The model under review builds one solid part; all positions refer to its coordinate system, in mm. Face numbers are marked on the shaded views. A direction names the side the tool comes from. Give positions to 0.01 mm unless a question says otherwise; leave off trailing zeros. Write each loop counter-clockwise with the first axis right and the second up, starting at its lowest first coordinate (ties: lowest second). Pieces come first, ordered by that corner, then holes. Notation, with made-up numbers: (64.25, 29.5) - (104.25, 29.5) arc R14 ccw to (104.25, 38.5) - close; hole circle Ø5 at (52, -27.5). An arc over 180 degrees is marked (long way). One line per question, with ' | ' between items. Start each with the question number.
```python
from build123d import *

# Parameters (mm, degrees)
SZKIC1_W                    = 40
SZKIC1_H                    = 20
SZKIC1_R                    = 2.25
DODANIE_WYCI_GNI_CIE1_DEPTH = 2
SZKIC3_W                    = 22
SZKIC3_H                    = 20
DODANIE_WYCI_GNI_CIE3_DEPTH = 3
ZAOKR_GLENIE1_R             = 3


with BuildPart() as part:
    # Szkic1 → Dodanie-wyciągnięcie1 (new body)
    with BuildSketch(Plane.XY):
        with Locations((0.494567618, 0.286392586)):
            Rectangle(SZKIC1_W, SZKIC1_H)
        with Locations((-9.505432382, 5.286392586)):
            Circle(SZKIC1_R, mode=Mode.SUBTRACT)
        with Locations((-9.505432382, -4.713607414)):
            Circle(SZKIC1_R, mode=Mode.SUBTRACT)
    extrude(amount=DODANIE_WYCI_GNI_CIE1_DEPTH)

    # Szkic3 → Dodanie-wyciągnięcie3 (add)
    with BuildSketch(Plane.XY.offset(2)):
        with Locations((9.494567618, 0.286392586)):
            Rectangle(SZKIC3_W, SZKIC3_H)
    extrude(amount=DODANIE_WYCI_GNI_CIE3_DEPTH)

    # Zaokrąglenie1
    zaokr_glenie1_edges = [part.edges().sort_by_distance(p)[0] for p in [
        (20.494567618, -9.713607414, 2.5),
        (-19.505432382, -9.713607414, 1),
        (-19.505432382, 10.286392586, 1),
        (20.494567618, 10.286392586, 2.5),
        (-1.505432382, 10.286392586, 3.5),
        (-1.505432382, -9.713607414, 3.5),
    ]]
    fillet(zaokr_glenie1_edges, radius=ZAOKR_GLENIE1_R)


solid = part.part
```
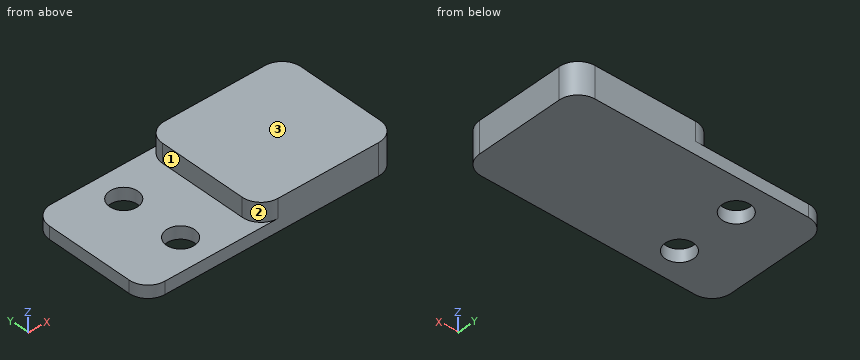
Item 1: Machinability: for the marked faces 1, 2 and 3, which of the approach directions +Z, -Z, +X, -X, +Y, -Y give a long, thin tool a straight path to every point of the face, cutting with its end or side? Answer none if there is none.
Item 2: Clearance check with flat-ended pins moving along their axes: P1, Ø10, axis at x = -8.5, y = 1, coming from the +Z side; P2, Ø2.5, axis at x = -9.51, y = 5.29, coming from the -Z side. State where each tip first meets the part, or that it passes through.
Item 3: Take a section at A-A (y = 5.75). Give the boundary of the cut face in (x, z), plus the area to 3 significant figures.
Item 4: Take a section at D-D (y = -1.5). Give the boundary of the cut face in (x, z).
Item 5: Take a section at C-C (x = -9). Give the boundary of the cut face in (y, z).
Item 6: Take a section at B-B (z = 1.25). Give the boundary of the cut face in (x, y).
Item 7: For probe 1 along Y at (x, z) = (-9, 1.25); probe 2 along Z at (x, y) = (-3, 3.75); probe 3 along X at (y, z) = (1.75, 3.05), list the stretches that pass through material, from the lowest coordinate up.
Check sheet entries:
1) face 1: +Z, -X, +Y, -Y | face 2: +Z, -X, -Y | face 3: +Z, +X, -X, +Y, -Y
2) P1: stops at z = 2 | P2: passes through
3) outline: (-19.51, 0) - (-11.71, 0) - (-11.71, 2) - (-19.51, 2) - close; (-7.3, 0) - (20.49, 0) - (20.49, 5) - (-1.51, 5) - (-1.51, 2) - (-7.3, 2) - close | area: 137 mm^2
4) outline: (-19.51, 0) - (20.49, 0) - (20.49, 5) - (-1.51, 5) - (-1.51, 2) - (-19.51, 2) - close
5) outline: (-9.71, 0) - (-6.91, 0) - (-6.91, 2) - (-9.71, 2) - close; (-2.52, 0) - (3.09, 0) - (3.09, 2) - (-2.52, 2) - close; (7.48, 0) - (10.29, 0) - (10.29, 2) - (7.48, 2) - close
6) outline: (-19.51, -6.71) arc R3 ccw to (-16.51, -9.71) - (17.49, -9.71) arc R3 ccw to (20.49, -6.71) - (20.49, 7.29) arc R3 ccw to (17.49, 10.29) - (-16.51, 10.29) arc R3 ccw to (-19.51, 7.29) - close; hole circle Ø4.5 at (-9.51, -4.71); hole circle Ø4.5 at (-9.51, 5.29)
7) probe 1: y = -9.71 to -6.91, -2.52 to 3.09, 7.48 to 10.29 | probe 2: z = 0 to 2 | probe 3: x = -1.51 to 20.49
